For this review, take the finished solid that the model builds, in its own axes (mm). A direction names the side the tool comes from. Give positions to 0.01 mm unless a question says otherwise; leave off trailing zeros. Order: outer loops, then holes, each group sorted by start corner. A loop starts at its lowest first (then second) coordinate and runs counter-clockwise, first axis right, second up. Notation, with made-up numbers: M -8,-36.75 L 33,-36.75 A29 ccw 33,-10.75 Z; hole C 79.5,-25 d4. An arc over 180 degrees is marked long. Answer as CSV lines item,"result". Start each with the question number.
1. We need section A-A, the plane y = -14.5. Give the boundary of the cut face in (x, z), and give its area (3 significant figures).
2. We need section D-D, the plane z = -15. Give the boundary of the cut face in (x, y).
3. We need section B-B, the plane z = -8.5. Give the boundary of the cut face in (x, y), and give its area (3 significant figures).
4. For line 1 along Y through (x, z) = (-41, 33); line 2 along X through (y, z) = (-13, 5); line 3 along Z through (x, y) = (-34.5, -12.5), list the stretches that pass through material, from the lowest coordinate up.
5. Mouldability with a two-part tool opening along X and no side actions: class faces 4 (the flat face through (-27.13, -12.73, -1.15)), 5 (the cylindrical face through (-14.299, -17.296, 2.661)), 6 (the flat face through (-32, 6, 37.259)), 7 (the flat face through (2.647, 6.261, 7.947)) as pulls with the +X half, pulls with the -X half, needs draft (parallel to the pull), parting line crosses it, or undercut.
6. Machinability: for faces 1 (the flat face through (-32, -13, 32.719)), 2 (the flat face through (-5, 0, 12)), 3 (the flat face through (-21, -25.4, -1)), which of the approach directions +Z, -Z, +X, -X, +Y, -Y give a long, thin tool a straight path to every point of the face, cutting with its end or side? Answer none if there is none.
7. Clearance check with flat-ended pins moving along their axes: P1, Ø10, axis at x = -20, y = -8, coming from the +Z side; P2, Ø1.5, axis at y = -11, z = 29.5, coming from the +X side; P3, Ø10, axis at y = 4.5, z = 10.5, coming from the +X side. State where each tip first meets the part, or that it passes through.
8. We need section C-C, the plane x = 12.5. Give the boundary of the cut face in (y, z), and give its area (3 significant figures).
from build123d import *

# Parameters (mm, degrees)
F0_W     = 93.299177
F0_H     = 54.989692
F1_DEPTH = 25.4
F3_DEPTH = 25.4
F4_R     = 5.858144
F5_DEPTH = 25.4
F6_W     = 80.10165
F6_H     = 55.35629
F7_DEPTH = 25.4
F9_DEPTH = 12.7


with BuildPart() as f1:
    # F0 (on Front) → F1 (new body)
    with BuildSketch(Plane.XZ):
        with Locations((2.107938, 5.224021)):
            Rectangle(F0_W, F0_H)
    extrude(amount=F1_DEPTH)

    # F2 (on face) → F3 (cut)
    with BuildSketch(Plane.XZ.offset(25.4)):
        Polygon((55.539589, 35.285052), (-18.513195, 32.718867), (16.313609, -22.270825), (61.221853, -24.653712), align=None)
    extrude(amount=-F3_DEPTH, mode=Mode.SUBTRACT)

    # F4 (on face) → F5 (cut)
    with BuildSketch(Plane(origin=(1.57643, 0, 0.998406), x_dir=(0, 1, 0), z_dir=(0.844819, 0, 0.535052))):
        with Locations((-12.647629, 13.463562)):
            Circle(F4_R)
    extrude(amount=-F5_DEPTH, mode=Mode.SUBTRACT)

    # F6 (on Front) → F7 (cut)
    with BuildSketch(Plane.XZ):
        with Locations((-4.857423, 5.040722)):
            Rectangle(F6_W, F6_H)
    extrude(amount=-F7_DEPTH, mode=Mode.SUBTRACT)

    # F8 (on face) → F9 (join)
    with BuildSketch(Plane(origin=(0, 0, 0), x_dir=(-1, 0, 0), z_dir=(0, 1, 0))):
        Polygon((44.54165, 37.259281), (18.513195, 37.259281), (-24.408791, -22.19771), (44.54165, -22.270825), align=None)
    extrude(amount=F9_DEPTH)


solid = f1.part
Result set:
1,outline,"M -44.54,-22.27 L 16.31,-22.27 L -2.65,7.68 L -24.11,-5.91 L -30.06,3.48 L -8.6,17.07 L -18.51,32.72 L -44.54,32.72 Z"
1,area,"2,110 mm2"
2,outline,"M -44.54,-25.4 L 11.71,-25.4 L 11.71,0 L 19.21,0 L 19.21,12.7 L -44.54,12.7 Z"
3,outline,"M -44.54,-25.4 L 7.59,-25.4 L 7.59,0 L 14.52,0 L 14.52,12.7 L -44.54,12.7 Z"
3,area,"2,070 mm2"
4,line 1,"0 to 12.7"
4,line 2,"-44.54 to -28.2, -6.34 to -0.96"
4,line 3,"-22.27 to 32.72"
5,face 4,"undercut"
5,face 5,"undercut"
5,face 6,"needs draft"
5,face 7,"pulls with the +X half"
6,face 1,"+Z, +X, -X, -Y"
6,face 2,"+Z, +X, -Y"
6,face 3,"+Z, -Z, +X, -X, -Y"
7,P1,"z = 32.72"
7,P2,"x = -16"
7,P3,"x = 4.41"
8,outline,"M -25.4,-22.27 L 0,-22.27 L 0,-22.21 L 12.7,-22.21 L 12.7,-5.7 L 0,-5.7 L 0,-16.25 L -25.4,-16.25 Z"
8,area,"363 mm2"
